Verification items for this drawing (mm, ordinates from the low corner). A direction names the side the tool comes from. Coordinates: 2 decimals unless noted, no trailing zeros. Loops run counter-clockwise (first coordinate to the right, second up) from the corner with the lowest first, then second, coordinate; pieces in that order, holes last. Notation, with made-up numbers: (14, 44) -> (28, 44) arc R22 cw to (28, 75) -> close; hole circle Ø2 at (2.5, 0.5). An arc over 180 degrees is marked (long way). Write item = value, one per line.
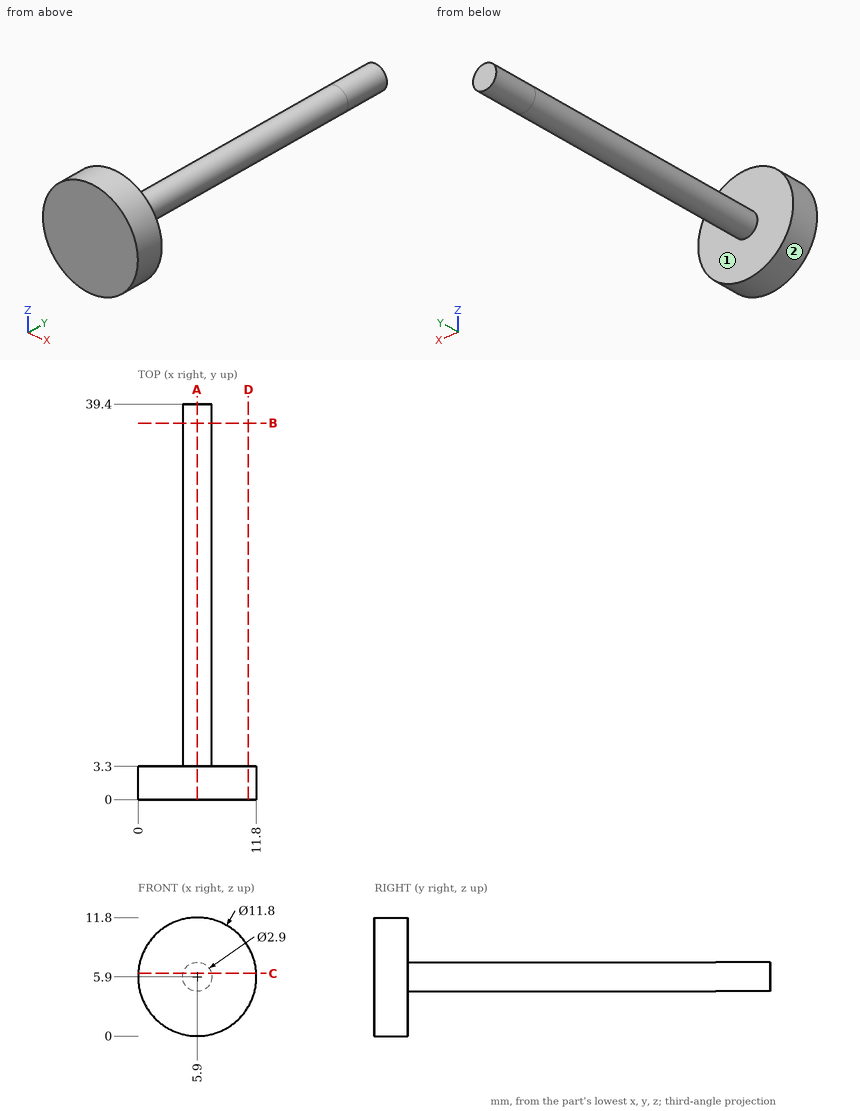
1) Sectioned sample at B-B, the plane y = 37.5. Record the cut outline in (x, z), plus the area to 3 significant figures.
Ans:
outline = circle Ø2.9 at (5.9, 5.9)
area = 6.61 mm2
2) Tool access check on the marked faces 1 and 2. Record the directions out of +Z, -Z, +X, -X, +Y, -Y that give a thin tool (end or side, any length) a straight path to the whole face; none if there is none.
Ans:
face_1 = +Y
face_2 = +Y, -Y
3) Sectioned sample at A-A, the plane x = 5.9. Record the cut outline in (y, z).
Ans:
outline = (0, 0) -> (3.3, 0) -> (3.3, 4.45) -> (39.4, 4.45) -> (39.4, 7.35) -> (3.3, 7.35) -> (3.3, 11.8) -> (0, 11.8) -> close
4) Material ranges on line 1 (Y direction, x = 9.5, z = 9.5); line 2 (Z direction, x = 6, y = 26); line 3 (X direction, y = 28, z = 5.75), recorded low to high.
Ans:
line_1 = 0 to 3.3
line_2 = 4.45 to 7.35
line_3 = 4.46 to 7.34
5) Sectioned sample at D-D, the plane x = 11. Record the cut outline in (y, z).
Ans:
outline = (0, 2.93) -> (3.3, 2.93) -> (3.3, 8.87) -> (0, 8.87) -> close
6) Sectioned sample at C-C, the plane z = 6.25. Record the cut outline in (x, y).
Ans:
outline = (0.01, 0) -> (11.79, 0) -> (11.79, 3.3) -> (7.31, 3.3) -> (7.31, 39.4) -> (4.49, 39.4) -> (4.49, 3.3) -> (0.01, 3.3) -> close
7) Depth check by flat-ended pin: pin 1 Ø3 at (x, y) = (4, 25.5) entering from +Z; pin 2 Ø5 at (y, z) = (22, 4) entering from +X; pin 3 Ø4 at (y, z) = (25, 6) entering from -X. Enter the tip coordinate at first touch or a pass-through.
Ans:
pin_1 = 7.29
pin_2 = 7.35
pin_3 = 4.45
